from build123d import *

# Parameters (mm, degrees)
F0_R     = 6
F1_DEPTH = 6.35


# Not quite as in the source:
# - a feature names something its author has since deleted; it is built from what else it names


with BuildPart() as f1:
    # F0 (on Top) → F1 (new body)
    with BuildSketch(Plane.XY):
        with BuildLine():
            Line((-27.5, 15), (-27.5, 7.5))
            Line((-27.5, 7.5), (-21.15, 7.5))
            Line((-21.15, 7.5), (-21.15, -7.5))
            Line((-21.15, -7.5), (-27.5, -7.5))
            Line((-27.5, -7.5), (-27.5, -15))
            Line((-27.5, -15), (3.27e-08, -15))
            ThreePointArc((3.27e-08, -15), (-15, -1.63e-08), (0, 15))
            Line((0, 15), (-27.5, 15))
        make_face()
        with BuildLine():
            ThreePointArc((15, 0), (10.6066017178, 10.6066017178), (0, 15))
            ThreePointArc((0, 15), (-15, -1.63e-08), (3.27e-08, -15))
            ThreePointArc((3.27e-08, -15), (10.6066017294, -10.6066017062), (15, 0))
        make_face()
        Circle(F0_R, mode=Mode.SUBTRACT)
    extrude(amount=F1_DEPTH)


solid = f1.part
Could you check a few things on this model? Use its own coordinates, in mm. A direction names the side the tool comes from. Coordinates: 2 decimals unless noted, no trailing zeros. Loops run counter-clockwise (first coordinate to the right, second up) from the corner with the lowest first, then second, coordinate; pieces in that order, holes last. Notation, with made-up numbers: (-22.75, 57) -> (-7.75, 57) arc R27 ccw to (-7.75, 80) -> close; hole circle Ø7 at (45, 34). An arc over 180 degrees is marked (long way). Answer in a Markdown table with one row per item.
(1) Imagine slicing it at D-D (y = 12.75). List the corners of the cut face in (x, z) for me, plus the area to 3 significant figures.
Results found:
| item | result |
|---|---|
| outline | (-27.5, 0) -> (7.9, 0) -> (7.9, 6.35) -> (-27.5, 6.35) -> close |
| area | 225 mm^2 |
(2) Imagine slicing it at A-A (y = 0). List the corners of the cut face in (x, z) for me, plus the area to 3 significant figures.
Results found:
| item | result |
|---|---|
| outline | (-21.15, 0) -> (-6, 0) -> (-6, 6.35) -> (-21.15, 6.35) -> close; (6, 0) -> (15, 0) -> (15, 6.35) -> (6, 6.35) -> close |
| area | 153 mm^2 |
(3) Will these pins go through, and if not, where does the flat tip stop? pin 1 Ø3 at (x, y) = (5.5, 4.5) entering from -Z; pin 2 Ø1 at (x, z) = (10, 4.5) entering from +Y.
Results found:
| item | result |
|---|---|
| pin 1 | stops at z = 0 |
| pin 2 | stops at y = 11.61 |
(4) Thinking about a two-plate mould opening in Y: for faces 1 (the face through (15, 0, 3)), 2 (the face through (-21.15, 0, 3)), 3 (the face through (-24, 7.5, 3)), 4 (the face through (-14, 15, 3)), which applies, released by +Y, released by -Y, zero draft, split by the parting line, or undercut?
Results found:
| item | result |
|---|---|
| face 1 | split by the parting line |
| face 2 | undercut |
| face 3 | undercut |
| face 4 | released by +Y |
(5) Imagine slicing it at B-B (x = 4). List the corners of the cut face in (y, z) for me.
Results found:
| item | result |
|---|---|
| outline | (-14.46, 0) -> (-4.47, 0) -> (-4.47, 6.35) -> (-14.46, 6.35) -> close; (4.47, 0) -> (14.46, 0) -> (14.46, 6.35) -> (4.47, 6.35) -> close |
(6) If I drill on probe 1 along Y at (x, z) = (-22.5, 2); probe 2 along X at (y, z) = (1, 6); probe 3 along X at (y, z) = (0.75, 1.25), over which ranges is the centre line in solid material (lowest first)?
Results found:
| item | result |
|---|---|
| probe 1 | y = -15 to -7.5, 7.5 to 15 |
| probe 2 | x = -21.15 to -5.92, 5.92 to 14.97 |
| probe 3 | x = -21.15 to -5.95, 5.95 to 14.98 |
(7) For faces 5 (the face through (-7, 0, 6.35)), 6 (the face through (-24, -7.5, 3)), which set-ups out of +Z, -Z, +X, -X, +Y, -Y let a thin tool reach every point of the face, with its end or its side?
Results found:
| item | result |
|---|---|
| face 5 | +Z, +X, -X, +Y, -Y |
| face 6 | +Z, -Z, -X |
(8) Imagine slicing it at C-C (z = 4.75). List the corners of the cut face in (x, y) for me.
Results found:
| item | result |
|---|---|
| outline | (-27.5, -15) -> (0, -15) arc R15 ccw to (0, 15) -> (-27.5, 15) -> (-27.5, 7.5) -> (-21.15, 7.5) -> (-21.15, -7.5) -> (-27.5, -7.5) -> close; hole circle Ø12 at (0, 0) |
